from build123d import *

# Parameters (mm, degrees)
BOSS_BORES_AND_POSITIVE_GEARBOX_MOUN_2_W       = 184
BOSS_BORES_AND_POSITIVE_GEARBOX_MOUN_2_H       = 42
BOSS_BORES_AND_POSITIVE_GEARBOX_MOUN_2_R       = 6.3
BOSS_BORES_AND_POSITIVE_GEARBOX_MOUN_2_R_2     = 1.7
BOSS_BORES_AND_POSITIVE_GEARBOX_MOUNTING_DEPTH = 1


with BuildPart() as part:
    # Boss bores and positive gearbox moun 2 → Boss bores and positive gearbox mounting (new body)
    with BuildSketch(Plane.XY):
        with Locations((0, 28)):
            Rectangle(BOSS_BORES_AND_POSITIVE_GEARBOX_MOUN_2_W, BOSS_BORES_AND_POSITIVE_GEARBOX_MOUN_2_H)
        with Locations((-62, 28.5)):
            Circle(BOSS_BORES_AND_POSITIVE_GEARBOX_MOUN_2_R, mode=Mode.SUBTRACT)
        with Locations((0, 28.5)):
            Circle(BOSS_BORES_AND_POSITIVE_GEARBOX_MOUN_2_R, mode=Mode.SUBTRACT)
        with Locations((62, 28.5)):
            Circle(BOSS_BORES_AND_POSITIVE_GEARBOX_MOUN_2_R, mode=Mode.SUBTRACT)
        with Locations((-52.5, 28.5)):
            Circle(BOSS_BORES_AND_POSITIVE_GEARBOX_MOUN_2_R_2, mode=Mode.SUBTRACT)
        with Locations((-60.25, 41.923393759)):
            Circle(BOSS_BORES_AND_POSITIVE_GEARBOX_MOUN_2_R_2, mode=Mode.SUBTRACT)
        with Locations((-75.75, 41.923393759)):
            Circle(BOSS_BORES_AND_POSITIVE_GEARBOX_MOUN_2_R_2, mode=Mode.SUBTRACT)
        with Locations((-83.5, 28.5)):
            Circle(BOSS_BORES_AND_POSITIVE_GEARBOX_MOUN_2_R_2, mode=Mode.SUBTRACT)
        with Locations((-75.75, 15.076606241)):
            Circle(BOSS_BORES_AND_POSITIVE_GEARBOX_MOUN_2_R_2, mode=Mode.SUBTRACT)
        with Locations((-60.25, 15.076606241)):
            Circle(BOSS_BORES_AND_POSITIVE_GEARBOX_MOUN_2_R_2, mode=Mode.SUBTRACT)
        with Locations((9.5, 28.5)):
            Circle(BOSS_BORES_AND_POSITIVE_GEARBOX_MOUN_2_R_2, mode=Mode.SUBTRACT)
        with Locations((1.75, 41.923393759)):
            Circle(BOSS_BORES_AND_POSITIVE_GEARBOX_MOUN_2_R_2, mode=Mode.SUBTRACT)
        with Locations((-13.75, 41.923393759)):
            Circle(BOSS_BORES_AND_POSITIVE_GEARBOX_MOUN_2_R_2, mode=Mode.SUBTRACT)
        with Locations((-21.5, 28.5)):
            Circle(BOSS_BORES_AND_POSITIVE_GEARBOX_MOUN_2_R_2, mode=Mode.SUBTRACT)
        with Locations((-13.75, 15.076606241)):
            Circle(BOSS_BORES_AND_POSITIVE_GEARBOX_MOUN_2_R_2, mode=Mode.SUBTRACT)
        with Locations((1.75, 15.076606241)):
            Circle(BOSS_BORES_AND_POSITIVE_GEARBOX_MOUN_2_R_2, mode=Mode.SUBTRACT)
        with Locations((71.5, 28.5)):
            Circle(BOSS_BORES_AND_POSITIVE_GEARBOX_MOUN_2_R_2, mode=Mode.SUBTRACT)
        with Locations((63.75, 41.923393759)):
            Circle(BOSS_BORES_AND_POSITIVE_GEARBOX_MOUN_2_R_2, mode=Mode.SUBTRACT)
        with Locations((48.25, 41.923393759)):
            Circle(BOSS_BORES_AND_POSITIVE_GEARBOX_MOUN_2_R_2, mode=Mode.SUBTRACT)
        with Locations((40.5, 28.5)):
            Circle(BOSS_BORES_AND_POSITIVE_GEARBOX_MOUN_2_R_2, mode=Mode.SUBTRACT)
        with Locations((48.25, 15.076606241)):
            Circle(BOSS_BORES_AND_POSITIVE_GEARBOX_MOUN_2_R_2, mode=Mode.SUBTRACT)
        with Locations((63.75, 15.076606241)):
            Circle(BOSS_BORES_AND_POSITIVE_GEARBOX_MOUN_2_R_2, mode=Mode.SUBTRACT)
    extrude(amount=BOSS_BORES_AND_POSITIVE_GEARBOX_MOUNTING_DEPTH)


solid = part.part
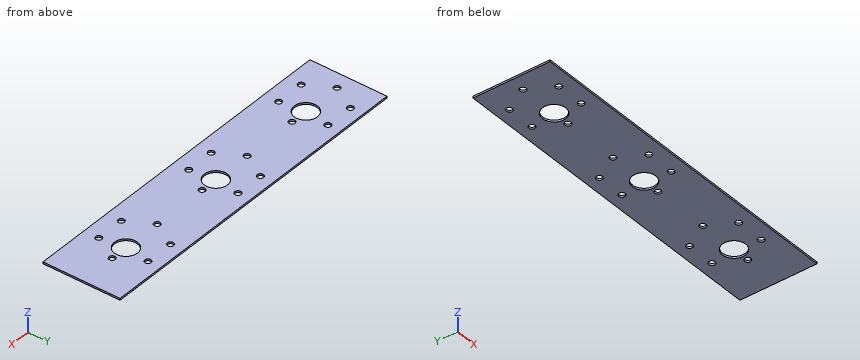
The model under review builds one solid part; all positions refer to its coordinate system, in mm. Give positions to 0.01 mm unless a question says otherwise; leave off trailing zeros. Order: outer loops, then holes, each group sorted by start corner. A loop starts at its lowest first (then second) coordinate and runs counter-clockwise, first axis right, second up. Notation, with made-up numbers: M 53,-5 L 108,-5 A19 ccw 108,12 Z; hole C 13,-32 d5. An arc over 180 degrees is marked long. Answer in a Markdown table with one row per item. Add a question column.
1. Add section B-B on x = 48.25. State the section outline as (y, z) points.
2. To check wall thickness, follow line 1 along Y through (x, z) = (48.25, 0.35); line 2 along X through (y, z) = (25, 0.25); line 3 along Y through (x, z) = (62, 0.2). State the ranges of each line that lie inside material, in increasing order.
3. Add section A-A on x = -21.5. State the section outline as (y, z) points, plus the area to 3 significant figures.
4. Add section D-D on z = 0.25. Count the separate pieces of the cut face and the enclosed holes in it, plus the area to 3 significant figures.
5. Add section C-C on y = 33. State the section outline as (x, z) points.
The answers:
| question | item | result |
|---|---|---|
| 1 | outline | M 7,0 L 13.38,0 L 13.38,1 L 7,1 Z; M 16.78,0 L 40.22,0 L 40.22,1 L 16.78,1 Z; M 43.62,0 L 49,0 L 49,1 L 43.62,1 Z |
| 2 | line 1 | 7 to 13.38, 16.78 to 40.22, 43.62 to 49 |
| 2 | line 2 | -92 to -67.24, -56.76 to -5.24, 5.24 to 56.76, 67.24 to 92 |
| 2 | line 3 | 7 to 22.2, 34.8 to 49 |
| 3 | outline | M 7,0 L 26.8,0 L 26.8,1 L 7,1 Z; M 30.2,0 L 49,0 L 49,1 L 30.2,1 Z |
| 3 | area | 38.6 mm2 |
| 4 | separate pieces | 1 |
| 4 | enclosed holes | 21 |
| 4 | area | 7,190 mm2 |
| 5 | outline | M -92,0 L -66.41,0 L -66.41,1 L -92,1 Z; M -57.59,0 L -4.41,0 L -4.41,1 L -57.59,1 Z; M 4.41,0 L 57.59,0 L 57.59,1 L 4.41,1 Z; M 66.41,0 L 92,0 L 92,1 L 66.41,1 Z |
